Can you work these out from the model? Positions are in its coordinate system, mm. Face numbers are marked on the shaded views. A direction names the side the tool comes from. Round coordinates to 2 decimals unless told otherwise and drop trailing zeros. Order: outer loops, then holes, each group sorted by start corner. A loop starts at its lowest first (then second) coordinate and runs counter-clockwise, first axis right, second up. Notation, with made-up numbers: M -9.5,-21.5 L 2.5,-21.5 A13 cw 2.5,2.5 Z; hole C -22.75,-38 d7. An arc over 180 degrees is marked long. One line per question, with ' | ' between items.
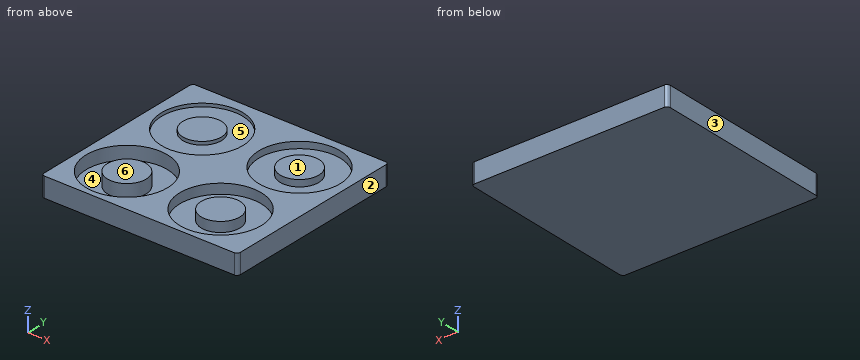
```python
from build123d import *

# Parameters (mm, degrees)
BOSS_EXTRUDE1_DEPTH   = 6
CAVITY1_START         = -3
CAVITY1_OUTLINE_R     = 12.36
CAVITY1_OUTLINE_R_2   = 5.8674
CAVITY1_DEPTH         = 3
CAVITY1_START_2       = -2
CAVITY1_2_OUTLINE_R   = 12.36
CAVITY1_2_OUTLINE_R_2 = 5.8674
CAVITY1_2_DEPTH       = 2
CAVITY1_START_3       = -4
CAVITY1_3_OUTLINE_R   = 12.36
CAVITY1_3_OUTLINE_R_2 = 5.8674
CAVITY1_3_DEPTH       = 1
CAVITY1_START_4       = -1
CAVITY1_4_OUTLINE_R   = 12.36
CAVITY1_4_OUTLINE_R_2 = 5.8674
CAVITY1_4_DEPTH       = 1


# Read off the part's stored shape, not the designer's step: Cavity1
with BuildPart() as part:
    # Sketch1 → Boss-Extrude1 (new body)
    with BuildSketch(Plane.XY):
        with BuildLine():
            Line((-14.454108138, 15.257956391), (43.072620808, 15.257956391))
            ThreePointArc((43.072620808, 15.257956391), (43.77972759, 14.965063172), (44.072620808, 14.257956391))
            Line((44.072620808, 14.257956391), (44.072620808, -39.722776706))
            ThreePointArc((44.072620808, -39.722776706), (43.77972759, -40.429883487), (43.072620808, -40.722776706))
            Line((43.072620808, -40.722776706), (-14.454108138, -40.722776706))
            ThreePointArc((-14.454108138, -40.722776706), (-15.16121492, -40.429883487), (-15.454108138, -39.722776706))
            Line((-15.454108138, -39.722776706), (-15.454108138, 14.257956391))
            ThreePointArc((-15.454108138, 14.257956391), (-15.16121492, 14.965063172), (-14.454108138, 15.257956391))
        make_face()
    extrude(amount=-BOSS_EXTRUDE1_DEPTH)

    # Cavity1 outline → Cavity1 (cut)
    # profile 1 of 2: a face of its own
    with BuildSketch(Plane.XY.offset(CAVITY1_START)):
        with Locations((-0.968104395, -26.708239151)):
            Circle(CAVITY1_OUTLINE_R)
        with Locations((-0.968104395, -26.708239151)):
            Circle(CAVITY1_OUTLINE_R_2, mode=Mode.SUBTRACT)
    # profile 2 of 2: a face of its own
    with BuildSketch(Plane.XY.offset(CAVITY1_START)):
        with Locations((27.453101021, -26.716944952)):
            Circle(CAVITY1_OUTLINE_R)
        with Locations((27.453101021, -26.716944952)):
            Circle(CAVITY1_OUTLINE_R_2, mode=Mode.SUBTRACT)
    extrude(amount=CAVITY1_DEPTH, mode=Mode.SUBTRACT)

    # Cavity1 2 outline → Cavity1 2 (cut)
    with BuildSketch(Plane.XY.offset(CAVITY1_START_2)):
        with Locations((29.157558022, 0.437297786)):
            Circle(CAVITY1_2_OUTLINE_R)
        with Locations((29.157558022, 0.437297786)):
            Circle(CAVITY1_2_OUTLINE_R_2, mode=Mode.SUBTRACT)
    extrude(amount=CAVITY1_2_DEPTH, mode=Mode.SUBTRACT)

    # Cavity1 3 outline → Cavity1 3 (cut)
    with BuildSketch(Plane.XY.offset(CAVITY1_START_3)):
        with Locations((-0.968104395, -26.708239151)):
            Circle(CAVITY1_3_OUTLINE_R)
        with Locations((-0.968104395, -26.708239151)):
            Circle(CAVITY1_3_OUTLINE_R_2, mode=Mode.SUBTRACT)
    extrude(amount=CAVITY1_3_DEPTH, mode=Mode.SUBTRACT)

    # Cavity1 4 outline → Cavity1 4 (cut)
    with BuildSketch(Plane.XY.offset(CAVITY1_START_4)):
        Circle(CAVITY1_4_OUTLINE_R)
        Circle(CAVITY1_4_OUTLINE_R_2, mode=Mode.SUBTRACT)
    extrude(amount=CAVITY1_4_DEPTH, mode=Mode.SUBTRACT)


solid = part.part
```
(1) Thinking about a two-plate mould opening in X: for the marked faces 1, 2, 3 and 4, which applies, released by +X, released by -X, zero draft, split by the parting line, or undercut?
Final values:
face 1: zero draft | face 2: released by +X | face 3: released by -X | face 4: undercut
(2) If we section it at B-B on y = -34: Please give me the cut outline in (x, z).
Final values:
outline: M -15.45,-6 L 44.07,-6 L 44.07,0 L 37.44,0 L 37.44,-3 L 17.47,-3 L 17.47,0 L 9.01,0 L 9.01,-4 L -10.95,-4 L -10.95,0 L -15.45,0 Z
(3) Please list where these lines run through material, in increasing order: probe 1 along Y at (x, z) = (1.5, -3.05); probe 2 along Y at (x, z) = (0, -0.2); probe 3 along Y at (x, z) = (2.5, -0.75). Write a range as [from, to].
Final values:
probe 1: [-40.72, -38.82], [-32.03, -21.39], [-14.6, 15.26] | probe 2: [-40.72, -39.03], [-32.5, -20.92], [-14.39, -12.36], [-5.87, 5.87], [12.36, 15.26] | probe 3: [-40.72, -38.57], [-31.44, -21.98], [-14.84, -12.1], [-5.31, 5.31], [12.1, 15.26]
(4) If we section it at D-D on x = 0: Please give me the cut outline in (y, z), plus the area to 3 significant figures.
Final values:
outline: M -40.72,-6 L 15.26,-6 L 15.26,0 L 12.36,0 L 12.36,-1 L 5.87,-1 L 5.87,0 L -5.87,0 L -5.87,-1 L -12.36,-1 L -12.36,0 L -14.39,0 L -14.39,-4 L -20.92,-4 L -20.92,0 L -32.5,0 L -32.5,-4 L -39.03,-4 L -39.03,0 L -40.72,0 Z | area: 271 mm^2
(5) If we section it at C-C on x = 28: Please give me the cut outline in (y, z), plus the area to 3 significant figures.
Final values:
outline: M -40.72,-6 L 15.26,-6 L 15.26,0 L 12.74,0 L 12.74,-2 L 6.19,-2 L 6.19,0 L -5.31,0 L -5.31,-2 L -11.87,-2 L -11.87,0 L -14.37,0 L -14.37,-3 L -20.88,-3 L -20.88,0 L -32.56,0 L -32.56,-3 L -39.06,-3 L -39.06,0 L -40.72,0 Z | area: 271 mm^2
(6) On a 3-axis mill with a long thin cutter (end or side, diameter ignored), from which of +Z, -Z, +X, -X, +Y, -Y can I reach the whole of each face in a straight line? I mean the marked faces 5 and 6. Say none if no direction works.
Final values:
face 5: +Z | face 6: +Z, +X, -X, +Y, -Y
(7) If we section it at A-A on x = 20.5: Please give me the cut outline in (y, z), plus the area to 3 significant figures.
Final values:
outline: M -40.72,-6 L 15.26,-6 L 15.26,0 L 9.26,0 L 9.26,-2 L -8.38,-2 L -8.38,0 L -16.5,0 L -16.5,-3 L -36.94,-3 L -36.94,0 L -40.72,0 Z | area: 239 mm^2
